Check sheet for the drawn part. Datum: minimum x, y, z corner. Units: mm. A direction names the side the tool comes from. Give positions to 0.01 mm unless a question says otherwise; leave off trailing zeros. Write each loop counter-clockwise with the first axis right and the second up, starting at its lowest first coordinate (ties: lowest second). Pieces come first, ordered by that corner, then holes. Notation, with made-up numbers: (32, 46) - (62, 46) arc R18 cw to (62, 50) - close; hole circle Ø6 at (78, 12.25). An arc over 180 degrees is marked (long way). One line per question, with ' | ' between items. Start each with the question number.
Q1. Thickness scan on L1, parallel to Z at x = 23, y = 3.5; L2, parallel to Y at x = 22.5, z = 1.95; L3, parallel to Y at x = 42, z = 3.3. Record the ranges inside material, lowest first. Write a range as [from, to].
Q2. Set-up check for the marked faces 1 and 2: record each of +Z, -Z, +X, -X, +Y, -Y from which the full face is reachable in a straight line by a thin tool's end or side.
Q3. Section check B-B on y = 9.25. Record the boundary of the cut face in (x, z), and give its area (3 significant figures).
Q4. Gauge pin test, flat ends, axial feed: P1, Ø0.8, axis at y = 0.5, z = 4.5, coming from the -X side; P2, Ø1, axis at y = 11, z = 4.5, coming from the -X side; P3, Ø1, axis at x = 44, y = 10, coming from the -Z side; P4, Ø0.5, axis at y = 0.5, z = 4.5, coming from the +X side. Record the tip position at first contact, or that the pin passes through.
Q5. Section check A-A on x = 26. Record the boundary of the cut face in (y, z).
Q6. Section check C-C on x = 18.5. Record the boundary of the cut face in (y, z), and give its area (4 significant figures).
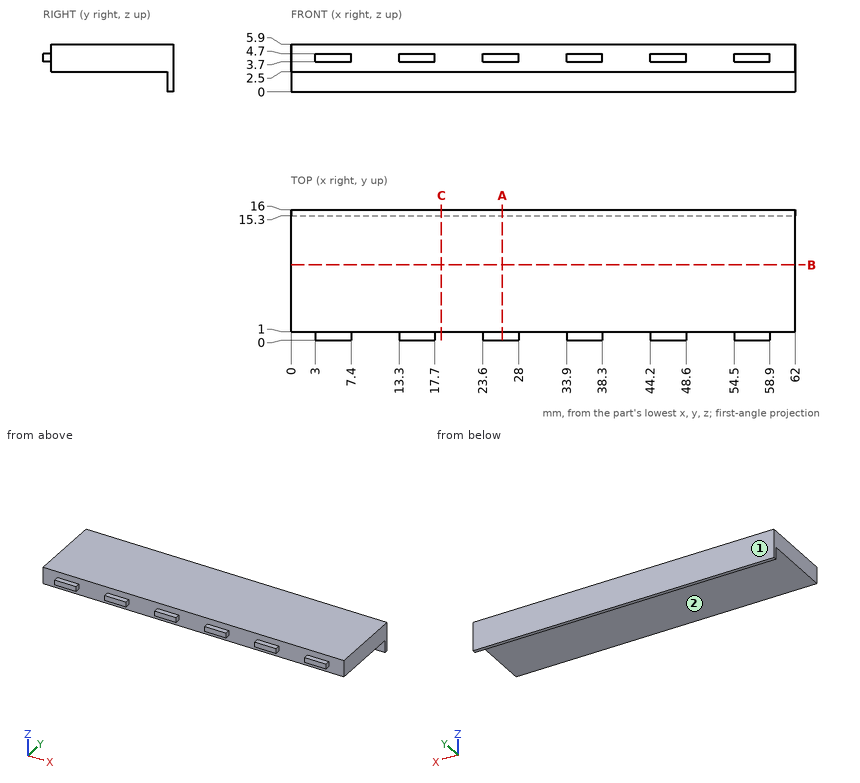
Working result:
1) L1: z = [2.5, 5.9] | L2: y = [15.3, 16] | L3: y = [1, 16]
2) face 1: +Z, -Z, +X, -X, +Y | face 2: -Z, +X, -X, -Y
3) outline: (0, 2.5) - (62, 2.5) - (62, 5.9) - (0, 5.9) - close | area: 211 mm2
4) P1: stops at x = 3 | P2: stops at x = 0 | P3: stops at z = 2.5 | P4: stops at x = 58.9
5) outline: (0, 3.7) - (1, 3.7) - (1, 2.5) - (15.3, 2.5) - (15.3, 0) - (16, 0) - (16, 5.9) - (1, 5.9) - (1, 4.7) - (0, 4.7) - close
6) outline: (1, 2.5) - (15.3, 2.5) - (15.3, 0) - (16, 0) - (16, 5.9) - (1, 5.9) - close | area: 52.75 mm2
